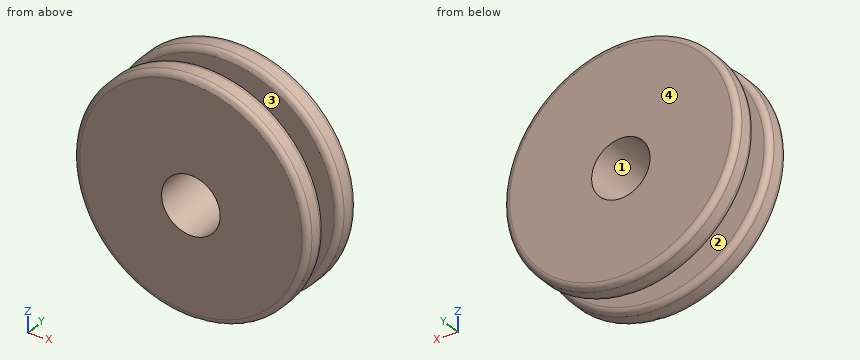
from build123d import *

# Parameters (mm, degrees)
F0_R     = 100
F1_DEPTH = 20
F2_R     = 60
F3_DEPTH = 20
F4_R     = 100
F5_DEPTH = 20
F6_R     = 25
F7_DEPTH = 100
F8_R     = 5


with BuildPart() as f1:
    # F0 (on Front) → F1 (new body)
    with BuildSketch(Plane.XZ):
        Circle(F0_R)
    extrude(amount=F1_DEPTH)

    # F2 (on face) → F3 (join)
    with BuildSketch(Plane.XZ.offset(20)):
        Circle(F2_R)
    extrude(amount=F3_DEPTH)

    # F4 (on face) → F5 (join)
    with BuildSketch(Plane.XZ.offset(40)):
        Circle(F4_R)
    extrude(amount=F5_DEPTH)

    # F6 (on face) → F7 (cut)
    with BuildSketch(Plane.XZ.offset(60)):
        with Locations((0, -5.704428)):
            Circle(F6_R)
    extrude(amount=-F7_DEPTH, mode=Mode.SUBTRACT)

    # F8
    f8_edges = [f1.edges().sort_by_distance(p)[0] for p in [
        (-100, -60, 0),
        (-100, -40, 0),
        (-100, -20, 0),
        (-100, 0, 0),
    ]]
    fillet(f8_edges, radius=F8_R)


solid = f1.part
Input: part model. Units: mm. Frame: model coordinates. Face numbers are marked on the shaded views. A direction names the side the tool comes from. Round coordinates to 2 decimals unless told otherwise and drop trailing zeros. Write each loop counter-clockwise with the first axis right and the second up, starting at its lowest first coordinate (ties: lowest second). Pieces come first, ordered by that corner, then holes.
1) Cut plane A-A (x = 0). Return the cut outline in (y, z), then the cut area to 3 significant figures.
2) Ray query, L1, parallel to Z at x = 0, y = -22.5; L2, parallel to Y at x = 64, z = 32; L3, parallel to X at y = -12.5, z = 6.5. Return the intervals inside material, ascending.
3) Draft query along Z for the marked faces 1 and 2. Return one class per face: pulls with the +Z half, pulls with the -Z half, needs draft (parallel to the pull), parting line crosses it, or undercut.
4) Cut plane B-B (z = 0). Return the cut outline in (x, y).
5) Reachability of the marked faces 3 and 4 from +Z, -Z, +X, -X, +Y, -Y: full face, straight path, thin tool, end or side. Return the list, or none.
6) Cut plane C-C (y = -8). Return the cut outline in (x, z).
7) Contact query for flat-ended pins moving along their axis: P1, Ø2, axis at y = -42, z = 3.5, coming from the +X side; P2, Ø1, axis at x = -46.5, y = -50, coming from the -Z side; P3, Ø4, axis at x = -47, y = -35, coming from the -Z side. Output: stop coordinate, or through.
Geometry says:
1. outline: (-60, -95) arc R5 ccw to (-55, -100) - (-45, -100) arc R5 ccw to (-40, -95) - (-40, -60) - (-20, -60) - (-20, -95) arc R5 ccw to (-15, -100) - (-5, -100) arc R5 ccw to (0, -95) - (0, -30.7) - (-60, -30.7) - close; (-60, 19.3) - (0, 19.3) - (0, 95) arc R5 ccw to (-5, 100) - (-15, 100) arc R5 ccw to (-20, 95) - (-20, 60) - (-40, 60) - (-40, 95) arc R5 ccw to (-45, 100) - (-55, 100) arc R5 ccw to (-60, 95) - close
1. area: 7,360 mm2
2. L1: z = -60 to -30.7, 19.3 to 60
2. L2: y = -60 to -40, -20 to 0
2. L3: x = -99.79 to -21.82, 21.82 to 99.79
3. face 1: undercut
3. face 2: needs draft
4. outline: (-100, -55) arc R5 ccw to (-95, -60) - (-24.34, -60) - (-24.34, 0) - (-95, 0) arc R5 ccw to (-100, -5) - (-100, -15) arc R5 ccw to (-95, -20) - (-60, -20) - (-60, -40) - (-95, -40) arc R5 ccw to (-100, -45) - close; (24.34, -60) - (95, -60) arc R5 ccw to (100, -55) - (100, -45) arc R5 ccw to (95, -40) - (60, -40) - (60, -20) - (95, -20) arc R5 ccw to (100, -15) - (100, -5) arc R5 ccw to (95, 0) - (24.34, 0) - close
5. face 3: none
5. face 4: +Z, -Z, +X, -X, +Y
6. outline: circle Ø200 at (0, 0); hole circle Ø50 at (0, -5.7)
7. P1: stops at x = 99.52
7. P2: stops at z = -88.79
7. P3: stops at z = -39.69
